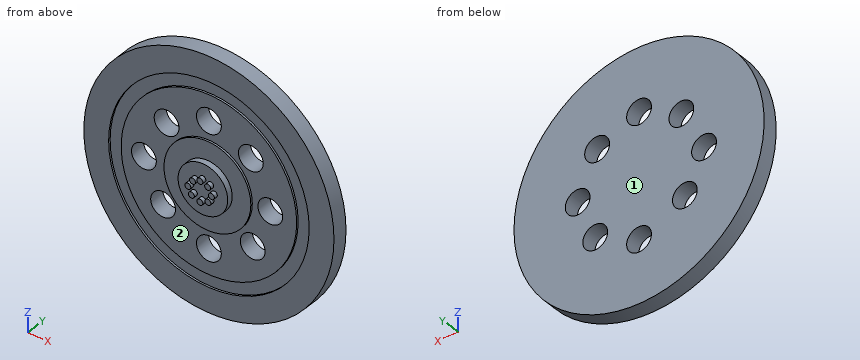
from build123d import *

# Parameters (mm, degrees)
F0_R      = 16.002
F1_DEPTH  = 2.032
F3_R      = 12.827
F3_R_2    = 11.2268
F4_DEPTH  = 0.254
F2_R      = 1.5875
F5_DEPTH  = 2.032
F6_R      = 5.55625
F7_DEPTH  = 0.254
F8_R      = 3.175
F9_DEPTH  = 0.762
F10_R     = 0.381
F11_DEPTH = 0.508


with BuildPart() as f1:
    # F0 (on Front) → F1 (new body)
    with BuildSketch(Plane.XZ):
        Circle(F0_R)
    extrude(amount=-F1_DEPTH)

    # F3 (on face) → F4 (cut)
    with BuildSketch(Plane.XZ):
        Circle(F3_R)
        Circle(F3_R_2, mode=Mode.SUBTRACT)
    extrude(amount=-F4_DEPTH, mode=Mode.SUBTRACT)

    # F2 (on face) → F5 (cut)
    with BuildSketch(Plane.XZ):
        with Locations((0, -7.9695228487)):
            Circle(F2_R)
        with Locations((-5.8604669757, -4.9584284425)):
            Circle(F2_R)
        with BuildLine():
            Line((-6.7264510825, 0), (-9.9014510825, 0))
            ThreePointArc((-9.9014510825, 0), (-8.3139510825, -1.5875), (-6.7264510825, 0))
        make_face()
        with BuildLine():
            ThreePointArc((-6.7264510825, 0), (-8.3139510825, 1.5875), (-9.9014510825, 0))
            Line((-9.9014510825, 0), (-6.7264510825, 0))
        make_face()
        with Locations((-5.4118158296, 5.3960969672)):
            Circle(F2_R)
        with Locations((0, 7.9223643988)):
            Circle(F2_R)
        with Locations((5.3672702052, 5.5701895617)):
            Circle(F2_R)
        with BuildLine():
            Line((6.2692415476, 0), (9.4442415476, 0))
            ThreePointArc((9.4442415476, 0), (7.8567415476, 1.5875), (6.2692415476, 0))
        make_face()
        with BuildLine():
            ThreePointArc((6.2692415476, 0), (7.8567415476, -1.5875), (9.4442415476, 0))
            Line((9.4442415476, 0), (6.2692415476, 0))
        make_face()
        with Locations((5.607039202, -5.3108036518)):
            Circle(F2_R)
    extrude(amount=-F5_DEPTH, mode=Mode.SUBTRACT)

    # F6 (on face) → F7 (join)
    with BuildSketch(Plane.XZ):
        Circle(F6_R)
    extrude(amount=F7_DEPTH)

    # F8 (on face) → F9 (join)
    with BuildSketch(Plane.XZ.offset(0.254)):
        Circle(F8_R)
    extrude(amount=F9_DEPTH)

    # F10 (on face) → F11 (join)
    with BuildSketch(Plane.XZ.offset(1.016)):
        with Locations((-1.543693963, 0)):
            Circle(F10_R)
        with Locations((-0.9479312136, 0.8902023229)):
            Circle(F10_R)
        with Locations((0, 1.2909881785)):
            Circle(F10_R)
        with Locations((0.9910054901, 0.9551946484)):
            Circle(F10_R)
        with Locations((1.4676158223, 0)):
            Circle(F10_R)
        with Locations((1.0343337624, -0.9079179104)):
            Circle(F10_R)
        with Locations((0, -1.3411998874)):
            Circle(F10_R)
        with Locations((-1.0887479328, -0.9079179104)):
            Circle(F10_R)
    extrude(amount=F11_DEPTH)


solid = f1.part
CAD build for the part. Positions are in the model's coordinates, mm. Face numbers are marked on the shaded views. A direction names the side the tool comes from. Coordinates: 2 decimals unless noted, no trailing zeros. Order: outer loops, then holes, each group sorted by start corner. A loop starts at its lowest first (then second) coordinate and runs counter-clockwise, first axis right, second up.
Item 1: 3-axis set-ups, long thin cutter, end or side, ignore diameter. For the marked faces 1 and 2: which of +Z, -Z, +X, -X, +Y, -Y reach the whole face in a straight line?
Check sheet entries:
face 1: +Z, -Z, +X, -X, +Y
face 2: -Y
Item 2: Drill centre lines: L1, parallel to Z at x = 0, y = 0.95; L2, parallel to X at y = 1.8, z = 5; L3, parallel to Z at x = 5.5, y = 1.8. Where is each one in solid material? Low to high.
Check sheet entries:
L1: z = -16 to -9.56, -6.38 to 6.33, 9.51 to 16
L2: x = -15.2 to -6.95, -3.87 to 3.89, 6.85 to 15.2
L3: z = -15.03 to -6.89, -3.73 to 3.99, 7.15 to 15.03
Item 3: Band-saw the part on A-A on y = 1. Give the number of separate pieces and of enclosed holes in the cut face, plus the area to 3 significant figures.
Check sheet entries:
separate pieces: 1
enclosed holes: 8
area: 741 mm2
Item 4: Pin check, flat tips, straight feed: pin 1 Ø2 at (x, y) = (9, 0.5) entering from -Z; pin 2 Ø3 at (x, z) = (-5.86, -4.96) entering from +Y; pin 3 Ø3.5 at (x, z) = (0, -7.97) entering from +Y; pin 4 Ø3.5 at (x, z) = (0, 7.92) entering from -Y. Stop position of each tip, or through.
Check sheet entries:
pin 1: stops at z = -13.86
pin 2: passes through
pin 3: stops at y = 2.03
pin 4: stops at y = 0
Item 5: Band-saw the part on C-C on z = -8.5. List the corners of the cut face in (x, y), plus the area to 3 significant figures.
Check sheet entries:
outline: (-13.56, 0) - (-9.61, 0) - (-9.61, 0.25) - (-7.33, 0.25) - (-7.33, 0) - (-1.5, 0) - (-1.5, 2.03) - (-13.56, 2.03) - close; (1.5, 0) - (7.33, 0) - (7.33, 0.25) - (9.61, 0.25) - (9.61, 0) - (13.56, 0) - (13.56, 2.03) - (1.5, 2.03) - close
area: 47.9 mm2
Item 6: Band-saw the part on B-B on x = 10. List the corners of the cut face in (y, z), plus the area to 3 significant figures.
Check sheet entries:
outline: (0, -12.49) - (2.03, -12.49) - (2.03, 12.49) - (0, 12.49) - (0, 8.03) - (0.25, 8.03) - (0.25, 5.1) - (0, 5.1) - (0, -5.1) - (0.25, -5.1) - (0.25, -8.03) - (0, -8.03) - close
area: 49.3 mm2
